from build123d import *

# Parameters (mm, degrees)
F0_W     = 296
F0_H     = 208
F0_R     = 4
F0_R_2   = 2.35
F0_R_3   = 18
F1_DEPTH = 8
F2_R     = 10


with BuildPart() as f1:
    # F0 (on Top) → F1 (new body)
    with BuildSketch(Plane.XY):
        Rectangle(F0_W, F0_H)
        with Locations((-123, -79)):
            Circle(F0_R, mode=Mode.SUBTRACT)
        with Locations((-27.5, -27.5)):
            Circle(F0_R_2, mode=Mode.SUBTRACT)
        with Locations((123, -79)):
            Circle(F0_R, mode=Mode.SUBTRACT)
        with Locations((27.5, -27.5)):
            Circle(F0_R_2, mode=Mode.SUBTRACT)
        with Locations((-27.5, 27.5)):
            Circle(F0_R_2, mode=Mode.SUBTRACT)
        with Locations((-123, 79)):
            Circle(F0_R, mode=Mode.SUBTRACT)
        Circle(F0_R_3, mode=Mode.SUBTRACT)
        with Locations((27.5, 27.5)):
            Circle(F0_R_2, mode=Mode.SUBTRACT)
        with Locations((123, 79)):
            Circle(F0_R, mode=Mode.SUBTRACT)
    extrude(amount=F1_DEPTH)

    # F2
    f2_edges = [f1.edges().sort_by_distance(p)[0] for p in [
        (-148, 104, 4),
        (-148, -104, 4),
        (148, -104, 4),
        (148, 104, 4),
    ]]
    fillet(f2_edges, radius=F2_R)


solid = f1.part
Geometry check sheet. Reference: the model listing, model coordinates, mm. Round coordinates to 2 decimals unless told otherwise and drop trailing zeros. Loops run counter-clockwise (first coordinate to the right, second up) from the corner with the lowest first, then second, coordinate; pieces in that order, holes last.
Item 1: Cross-section at A-A on y = 79. Record the boundary of the cut face in (x, z), then the cut area to 3 significant figures.
Item 2: Thickness scan on line 1 (Y direction, x = 123, z = 6); line 2 (X direction, y = 27, z = 2.75); line 3 (Y direction, x = -27.5, z = 5). Record the ranges inside material, lowest first.
Item 3: Cross-section at B-B on x = 0. Record the boundary of the cut face in (y, z).
Item 4: Gauge pin test, flat end, axial feed: pin 1 (6.5 mm diameter, centred on x = -123, y = 79, fed in from +Z). Record the tip position at first contact, or that the pin passes through.
Item 5: Cross-section at D-D on x = 123. Record the boundary of the cut face in (y, z), then the cut area to 3 significant figures.
Item 6: Cross-section at C-C on z = 5. Count the separate pieces of the cut face and the enclosed holes in it, then the cut area to 3 significant figures.
Item 7: Mould release check, pull along X, two halves, no side actions. Record for faces 1 (the cylindrical face through (144.99, -101.15, 4.06)), 2 (the flat face through (-2, 25, 8)), 3 (the cylindrical face through (122.133, -82.905, 3.944)): pulls with the +X half, pulls with the -X half, needs draft (parallel to the pull), parting line crosses it, or undercut.
Answer sheet:
1. outline: (-148, 0) - (-127, 0) - (-127, 8) - (-148, 8) - close; (-119, 0) - (119, 0) - (119, 8) - (-119, 8) - close; (127, 0) - (148, 0) - (148, 8) - (127, 8) - close
1. area: 2,240 mm2
2. line 1: y = -104 to -83, -75 to 75, 83 to 104
2. line 2: x = -148 to -29.8, -25.2 to 25.2, 29.8 to 148
2. line 3: y = -104 to -29.85, -25.15 to 25.15, 29.85 to 104
3. outline: (-104, 0) - (-18, 0) - (-18, 8) - (-104, 8) - close; (18, 0) - (104, 0) - (104, 8) - (18, 8) - close
4. pin 1: passes through
5. outline: (-104, 0) - (-83, 0) - (-83, 8) - (-104, 8) - close; (-75, 0) - (75, 0) - (75, 8) - (-75, 8) - close; (83, 0) - (104, 0) - (104, 8) - (83, 8) - close
5. area: 1,540 mm2
6. separate pieces: 1
6. enclosed holes: 9
6. area: 60,200 mm2
7. face 1: pulls with the +X half
7. face 2: needs draft
7. face 3: undercut
